Autodesk Inventor part; units mm, degrees
ref_plane "YZ Plane" through (0, 0, 0) normal (1, 0, 0) x (0, 1, 0)
ref_plane "XZ Plane" through (0, 0, 0) normal (0, 1, 0) x (-1, 0, 0)
ref_plane "XY Plane" through (0, 0, 0) normal (0, 0, 1) x (1, 0, 0)
sketch "Sketch2" plane through (0, 0, 0) normal (0, 1, 0) x (-1, 0, 0)
  circle A0 centre (0, 0) radius 14
  circle A1 centre (0, 0) radius 13
  dimension "d0" = 28
  dimension "d110" = 26
extrude "Extrusion1" add sketch "Sketch2" along normal blind 2 contours A0 | A1
sketch "Sketch13" plane through (0, 2, 0) normal (0, 1, 0) x (1, 0, 0)
  line L0 (0, 0) -> (8.8, 0)
  line L1 (8.8, 0) -> (8.8, -8.8)
  line L2 (8.8, -8.8) -> (-8.8, -8.8)
  line L3 (-8.8, -8.8) -> (-8.8, 8.8)
  line L4 (-8.8, 8.8) -> (8.8, 8.8)
  line L5 (8.8, 8.8) -> (8.8, 0)
  line L6 (0, 0) -> (8, 0)
  line L7 (8, 0) -> (8, -8)
  line L8 (8, -8) -> (-8, -8)
  line L9 (-8, -8) -> (-8, 8)
  line L10 (-8, 8) -> (8, 8)
  line L11 (8, 8) -> (8, 0)
  line L12 (-8.8, 0) -> (-8, 0)
  dimension "d104" = 8.8
  dimension "d105" = 8.8
  dimension "d106" = 17.6
  dimension "d107" = 17.6
  dimension "d108" = 17.6
  dimension "d109" = 8.8
  dimension "d114" = 8
  dimension "d115" = 8
  dimension "d116" = 16
  dimension "d117" = 16
  dimension "d118" = 16
  dimension "d119" = 8
extrude "Extrusion8" add sketch "Sketch13" along normal blind 6
shell "Shell2" thickness 0.8 removed faces 1 at (-2.9333, 8, -2.9333)
sketch "Sketch14" plane through (-8.8, 2, -8.8) normal (-1, 0, 0) x (0, 0, 1)
  line L0 (17.6, 6) -> (0, 6)
  line L1 (8.8, 6) -> (8.8, 3)
  line L2 (8.8, 3) -> (0, 3)
  line L3 (0, 0) -> (0, 6)
  circle A0 centre (8.8, 3) radius 0.5
  point P0 (8.8, -2)
  dimension "d121" = 3
  dimension "d122" = 8.8
  dimension "d123" = 1
hole "Hole5" at (-8.8, 5, 0) direction (1, 0, 0) diameter 1 depth 20
sketch "Sketch15" plane through (0, 2, 0) normal (0, 1, 0) x (1, 0, 0)
  line L0 (-8.8, -8.8) -> (8.8, -8.8)
  circle A0 centre (0, 0) radius 14
  line L1 (0, -8.8) -> (1.5, -8.8)
  line L2 (1.5, -8.8) -> (1.5, -14.8)
  line L3 (1.5, -14.8) -> (-1.5, -14.8)
  line L4 (1.5, -14.8) -> (4.5, -14.8) construction
  line L5 (-1.5, -14.8) -> (-1.5, -8.8)
  line L6 (-1.5, -8.8) -> (1.5, -8.8)
  point P0 (-1.5, -13.9194)
  point P1 (1.5, -13.9194)
  dimension "d132" = 1.5
  dimension "d133" = 6
  dimension "d134" = 3
  dimension "d136" = 6
  dimension "d137" = 3
extrude "Extrusion9" add sketch "Sketch15" along normal blind 6 contours L0 L2 A0 L5 picked at (0.667, -10.5303)
sketch "Sketch17" plane through (0, 2, 0) normal (0, 1, 0) x (1, 0, 0)
  circle A0 centre (0, 0) radius 14
  line L0 (0, 14) -> (-1.5, 14)
  line L1 (-1.5, 14) -> (-1.5, 8.8)
  line L2 (8.8, 8.8) -> (-8.8, 8.8)
  line L3 (-1.5, 8.8) -> (1.5, 8.8)
  line L4 (1.5, 8.8) -> (1.5, 14)
  line L5 (1.5, 14) -> (0, 14)
  point P0 (1.5, 8.8)
  point P1 (1.5, 13.9194)
  point P2 (-1.5, 13.9194)
  dimension "d159" = 1.5
  dimension "d160" = 3
extrude "Extrusion11" add sketch "Sketch17" along normal blind 6 contours L4 L2 L1 A0 picked at (0, 10.5333)
properties part number "Part6_containter_bottom" material "ABS Plastic"
CAD build for the part. Positions are in the model's coordinates, mm. A direction names the side the tool comes from. Give positions to 0.01 mm unless a question says otherwise; leave off trailing zeros. Write each loop counter-clockwise with the first axis right and the second up, starting at its lowest first coordinate (ties: lowest second). Pieces come first, ordered by that corner, then holes. Notation, with made-up numbers: M 54,50 L 91,50 A21 cw 91,85 Z; hole C 31.5,-12 d7. An arc over 180 degrees is marked long. Put each result on its own line as item: value. Start each with the question number.
(1) Probe L1, parallel to Y at x = -8.5, z = 0; L2, parallel to Z at x = -4, y = 5.5; L3, parallel to Z at x = 8.2, y = 5. List the from-to ranges inside material, lowest first.
(2) Flat gauge pins, fed straight in: pin 1 Ø4 at (x, y) = (4, 4.5) entering from -Z; pin 2 Ø3 at (y, z) = (6, 3) entering from -X; pin 3 Ø2.5 at (y, z) = (5.5, 11.5) entering from -X. Where does each tip first touch, or does it go through?
(3) Which spindle directions (+Z, -Z, +X, -X, +Y, -Y) get a long thin tool onto all of the face, cutting with end or side? Do faces 1 (the face through (8.8, 6, 0)), 2 (the face through (8, 4, 0)), 3 (the face through (-8.8, 6, 0)), 4 (the face through (-5, 5, -8.8)), 5 (the face through (5, 5, -8.8)). Say none if no direction does.
(4) Mould opens along X. For faces 6 (the face through (-5, 5, 8.8)), 7 (the face through (0, 5, 8)), 8 (the face through (-13.928, 1.315, -1.421)) say: +X half, -X half, draft (parallel to the pull), parting line (faces both ways), or undercut.
(5) Band-saw the part on B-B, the plane y = 6.5. Write the cut outline in (x, z).
(6) Band-saw the part on D-D, the plane y = 5. Write the cut outline in (x, z), and give its area (3 significant figures).
(7) Band-saw the part on A-A, the plane z = 0. Write the cut outline in (x, y), and give its area (3 significant figures).
(8) Band-saw the part on C-C, the plane x = 0. Write the cut outline in (y, z), and give its area (3 significant figures).
Response values:
1. L1: y = 0 to 0.8, 1.2 to 4.5, 5.5 to 8
1. L2: z = -8.8 to -8, 8 to 8.8
1. L3: z = -8.8 to -0.5, 0.5 to 8.8
2. pin 1: stops at z = -8.8
2. pin 2: stops at x = -8.8
2. pin 3: stops at x = -1.5
3. face 1: +Z, -Z, +X, +Y
3. face 2: +Y
3. face 3: +Z, -Z, -X, +Y
3. face 4: -Z, -X, +Y
3. face 5: -Z, +X, +Y
4. face 6: draft
4. face 7: undercut
4. face 8: parting line
5. outline: M -8.8,-8.8 L -1.5,-8.8 L -1.5,-13.92 A14 ccw 1.5,-13.92 L 1.5,-8.8 L 8.8,-8.8 L 8.8,8.8 L 1.5,8.8 L 1.5,13.92 A14 ccw -1.5,13.92 L -1.5,8.8 L -8.8,8.8 Z; hole M -8,-8 L 8,-8 L 8,8 L -8,8 Z
6. outline: M -8.8,-8.8 L -1.5,-8.8 L -1.5,-13.92 A14 ccw 1.5,-13.92 L 1.5,-8.8 L 8.8,-8.8 L 8.8,-0.5 L 8,-0.5 L 8,-8 L -8,-8 L -8,-0.5 L -8.8,-0.5 Z; M -8.8,0.5 L -8,0.5 L -8,8 L 8,8 L 8,0.5 L 8.8,0.5 L 8.8,8.8 L 1.5,8.8 L 1.5,13.92 A14 ccw -1.5,13.92 L -1.5,8.8 L -8.8,8.8 Z
6. area: 83.2 mm2
7. outline: M -14,0 L 14,0 L 14,2 L 8.8,2 L 8.8,4.5 L 8,4.5 L 8,1.2 L 13.2,1.2 L 13.2,0.8 L -13.2,0.8 L -13.2,1.2 L -8,1.2 L -8,4.5 L -8.8,4.5 L -8.8,2 L -14,2 Z; M -8.8,5.5 L -8,5.5 L -8,8 L -8.8,8 Z; M 8,5.5 L 8.8,5.5 L 8.8,8 L 8,8 Z
7. area: 40.6 mm2
8. outline: M 0,-14 L 8,-14 L 8,-8 L 1.2,-8 L 1.2,-13.2 L 0.8,-13.2 L 0.8,13.2 L 1.2,13.2 L 1.2,8 L 8,8 L 8,14 L 0,14 Z
8. area: 105 mm2
